Read the model definition and answer for the solid it produces. Units are mm, in the model's axes. Face numbers are marked on the shaded views. A direction names the side the tool comes from. Coordinates: 2 decimals unless noted, no trailing zeros. Write each loop counter-clockwise with the first axis right and the second up, starting at its lowest first coordinate (ties: lowest second). Pieces come first, ordered by that corner, then holes.
1) Find the intervals of material crossed by line 1 (X direction, y = 1.3, z = 40); line 2 (Z direction, x = 14.5, y = -26.5); line 3 (X direction, y = -19, z = -13), in increasing order.
2) The part is cut by section A-A (y = -37.5). Determine the outline of the cut face in (x, z).
3) The part is cut by section C-C (z = 9). Determine the outline of the cut face in (x, y), then the cut area to 3 significant figures.
4) The part is cut by section D-D (z = 18). Determine the outline of the cut face in (x, y), then the cut area to 3 significant figures.
5) Each of these flat-tipped pins is pushed along its axis until it touches: pin 1 Ø23 at (y, z) = (-34.5, -18) entering from -X; pin 2 Ø25 at (x, y) = (33, -26.5) entering from +Z; pin 3 Ø13.5 at (x, z) = (25, 24.5) entering from -Y; pin 4 Ø1.5 at (x, z) = (24.5, 1.5) entering from -Y. Where does it stop, or does it pass through?
6) Determine the mould class of the marked faces 1, 2, 3 and 4 for opening direction Z: +Z half, -Z half, draft (parallel to the pull), parting line (faces both ways), or undercut.
7) Which of the six approach directions +Z, -Z, +X, -X, +Y, -Y give full straight-line access (tool end or side, diameter ignored) to the marked faces 5, 6, 7 and 8?
8) The part is cut by section B-B (x = 25). Determine the outline of the cut face in (y, z), then the cut area to 3 significant figures.
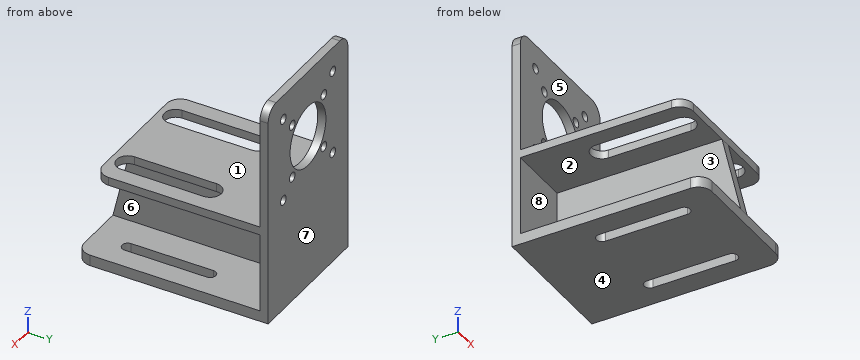
Autodesk Fusion 360 part; units mm, degrees
sketch "Sketch1" plane through (0, 0, 0) normal (0, 1, 0) x (1, 0, 0)
  line L0 (0, 0) -> (50, 0)
  line L1 (50, 0) -> (50, -49)
  line L2 (50, -49) -> (0, -49)
  line L3 (0, -49) -> (0, 0)
  line L4 (0, -24.5) -> (50, -24.5) construction
  line L5 (25, -49) -> (25, 0) construction
  circle A0 centre (25, -24.5) radius 11.25
  circle A1 centre (25, -24.5) radius 14 construction
  line L6 (0, -49) -> (0, -40) construction
  line L7 (0, -40) -> (9.5, -40) construction
  circle A2 centre (9.5, -40) radius 1.75
  line L8 (9.5, -40) -> (25, -24.5) construction
  circle A3 centre (15.1005, -34.3995) radius 1.75
  circle A4 centre (40.5, -40) radius 1.75
  circle A5 centre (34.8995, -34.3995) radius 1.75
  circle A6 centre (40.5, -9) radius 1.75
  circle A7 centre (34.8995, -14.6005) radius 1.75
  circle A8 centre (15.1005, -14.6005) radius 1.75
  circle A9 centre (9.5, -9) radius 1.75
  line L9 (0, -49) -> (5, -49)
  line L10 (5, -49) -> (5, -44) construction
  line L11 (5, -44) -> (0, -44) construction
  line L12 (0, -44) -> (0, -49)
  arc A10 (0, -44) -> (5, -49) centre (5, -44) ccw
  arc A11 (45, -49) -> (50, -44) centre (45, -44) ccw
  dimension "d1" = 50
  dimension "d2" = 49
  dimension "d3" = 22.5
  dimension "d4" = 28
  dimension "d5" = 9
  dimension "d6" = 9.5
  dimension "d7" = 3.5
  dimension "d8" = 3.5
  dimension "d11" = 5
  dimension "d12" = 5
extrude "Extrude2" add sketch "Sketch1" along normal blind 3 contours L0 L1 L2 L3 A10 A11
sketch "Sketch2" plane through (0, 0, 0) normal (0, 0, 1) x (1, 0, 0)
  line L0 (0, 3) -> (50, 3)
  line L1 (50, 3) -> (50, -67)
  line L2 (50, -67) -> (0, -67)
  line L3 (0, -67) -> (0, 3)
  line L4 (25, -67) -> (25, 3) construction
  line L5 (0, -67) -> (10, -67) construction
  line L6 (10, -67) -> (10, -54) construction
  line L7 (10, -54) -> (7.9, -54) construction
  line L8 (7.9, -54) -> (12.1, -54)
  line L9 (12.1, -54) -> (12.1, -24)
  line L10 (12.1, -24) -> (7.9, -24)
  line L11 (7.9, -24) -> (7.9, -54)
  arc A0 (7.9, -54) -> (12.1, -54) centre (10, -54) ccw
  arc A1 (12.1, -24) -> (7.9, -24) centre (10, -24) ccw
  arc A2 (37.9, -54) -> (42.1, -54) centre (40, -54) ccw
  line L12 (37.9, -54) -> (37.9, -24)
  line L13 (42.1, -24) -> (42.1, -54)
  arc A3 (42.1, -24) -> (37.9, -24) centre (40, -24) ccw
  line L14 (0, 0) -> (50, 0)
  point P0 (0, 3)
  dimension "d15" = 70
  dimension "d16" = 10
  dimension "d17" = 13
  dimension "d18" = 2.1
  dimension "d19" = 4.2
  dimension "d20" = 30
extrude "Extrude6" add sketch "Sketch2" against normal blind 32.6
extrude "Extrude7" cut sketch "Sketch2" against normal blind 28.6 contours L1 L2 L3 L14
ref_plane "WorkPlane1" through (25, -32, 5.7) normal (1, 0, 0) x (0, 0, -1)
sketch "Sketch6" plane through (25, -32, 5.7) normal (1, 0, 0) x (0, 1, 0)
  line L0 (32, -34.3) -> (-35, -34.3)
  line L1 (-35, -34.3) -> (-35, -5.3)
  line L2 (-35, -5.3) -> (32, -5.3)
  line L3 (32, -5.3) -> (32, -34.3)
  point P0 (32, -34.3)
  dimension "d48" = 67
  dimension "d49" = 29
sketch "Sketch10" plane through (0, 0, 0) normal (0, -1, 0) x (1, 0, 0)
  circle A0 centre (25, 24.5) radius 11.25
  circle A1 centre (9.5, 40) radius 1.75
  circle A2 centre (40.5, 40) radius 1.75
  circle A3 centre (15.1005, 34.3995) radius 1.75
  circle A4 centre (34.8995, 34.3995) radius 1.75
  circle A5 centre (40.5, 9) radius 1.75
  circle A6 centre (34.8995, 14.6005) radius 1.75
  circle A7 centre (15.1005, 14.6005) radius 1.75
  circle A8 centre (9.5, 9) radius 1.75
  arc A9 (5, 49) -> (0, 44) centre (5, 44) ccw
  line L0 (0, 44) -> (0, -28.6)
  line L1 (0, -28.6) -> (50, -28.6)
  line L2 (50, -28.6) -> (50, 44)
  arc A10 (50, 44) -> (45, 49) centre (45, 44) ccw
  line L3 (45, 49) -> (5, 49)
  line L4 (25, 24.5) -> (25, 3.4) construction
  dimension "d71" = 21.1
extrude "Extrude15" add sketch "Sketch6" along normal blind 2 and the other way blind 2
sketch "Sketch11" plane through (0, 0, 0.4) normal (0, 0, 1) x (-1, 0, 0)
  line L0 (-23, 67) -> (-27, 67)
  line L1 (-27, 67) -> (-27, 0)
  line L2 (-27, 0) -> (-23, 0)
  line L3 (-23, 0) -> (-23, 67)
  line L4 (0, 0) -> (-50, 0)
  line L5 (-50, 0) -> (-50, 60.1926)
  line L6 (-50, 60.1926) -> (0, 60.1926)
  line L7 (0, 60.1926) -> (0, 0)
  line L8 (-50, -3) -> (-50, 67)
  line L9 (-7.9, 24) -> (-5.9, 24)
  line L10 (-5.9, 24) -> (-14.1, 24)
  line L11 (-14.1, 24) -> (-14.1, 54)
  line L12 (-14.1, 54) -> (-5.9, 54)
  line L13 (-5.9, 54) -> (-5.9, 24)
  arc A0 (-5.9, 54) -> (-14.1, 54) centre (-10, 54) ccw
  arc A1 (-14.1, 24) -> (-5.9, 24) centre (-10, 24) ccw
  line L14 (-25, 67) -> (-25, 0)
  line L15 (-25, 60.1926) -> (-25, 53.1429)
  line L16 (-35.9, 24) -> (-35.9, 54)
  line L17 (-44.1, 54) -> (-44.1, 24)
  arc A2 (-35.9, 54) -> (-44.1, 54) centre (-40, 54) ccw
  arc A3 (-44.1, 24) -> (-35.9, 24) centre (-40, 24) ccw
  point P0 (-7.9, 24)
  dimension "d76" = 2
  dimension "d77" = 8.2
extrude "Extrude16" add sketch "Sketch11" along normal blind 3 contours L3 L4 L6 L7 | L2 L3 L4 L6 L14 L15 | L1 L2 L4 L6 L14 L15 | L1 L4 L5 L6 L8
sketch "Sketch12" plane through (27, 0, 0) normal (1, 0, 0) x (0, 1, 0)
  line L0 (0, 0.4) -> (-60.1926, 0.4)
  line L1 (-60.1926, 0.4) -> (-67, 0.4)
  line L2 (-67, 0.4) -> (-67, -28.6)
  line L3 (-67, -28.6) -> (0, -28.6)
  line L4 (0, -28.6) -> (0, 0.4)
  line L5 (-60.1926, 0.4) -> (-67, -28.6)
  line L6 (-67, 0.4) -> (-60.1926, 0.4)
extrude "Extrude17" cut sketch "Sketch12" against normal blind 8 contours L1 L2 L5 L6
fillet "Fillet3" radius 5 4 edges at (0, -60.1926, 1.9) (0, -67, -30.6) (50, -67, -30.6) (50, -60.1926, 1.9)
Reported:
1. line 1: x = 0 to 7.75, 11.25 to 38.75, 42.25 to 50
1. line 2: z = -32.6 to -28.6, 0.4 to 3.4
1. line 3: x = 23 to 27
2. outline: (0, -32.6) - (7.9, -32.6) - (7.9, -28.6) - (0, -28.6) - close; (0, 0.4) - (5.9, 0.4) - (5.9, 3.4) - (0, 3.4) - close; (12.1, -32.6) - (37.9, -32.6) - (37.9, -28.6) - (27, -28.6) - (27, 0.4) - (35.9, 0.4) - (35.9, 3.4) - (14.1, 3.4) - (14.1, 0.4) - (23, 0.4) - (23, -28.6) - (12.1, -28.6) - close; (42.1, -32.6) - (50, -32.6) - (50, -28.6) - (42.1, -28.6) - close; (44.1, 0.4) - (50, 0.4) - (50, 3.4) - (44.1, 3.4) - close
3. outline: (0, 0) - (7.75, 0) - (7.75, 3) - (0, 3) - close; (11.25, 0) - (38.75, 0) - (38.75, 3) - (11.25, 3) - close; (42.25, 0) - (50, 0) - (50, 3) - (42.25, 3) - close
3. area: 129 mm2
4. outline: (0, 0) - (15.82, 0) - (15.82, 3) - (0, 3) - close; (34.18, 0) - (50, 0) - (50, 3) - (34.18, 3) - close
4. area: 94.9 mm2
5. pin 1: stops at x = 0
5. pin 2: stops at z = 3.4
5. pin 3: passes through
5. pin 4: stops at y = -60.19
6. face 1: +Z half
6. face 2: undercut
6. face 3: undercut
6. face 4: -Z half
7. face 5: +Z, +X, -X, -Y
7. face 6: +X, -Y
7. face 7: +Z, -Z, +X, -X, +Y
7. face 8: -X, -Y
8. outline: (-67, -32.6) - (3, -32.6) - (3, 13.25) - (0, 13.25) - (0, 3.4) - (-60.19, 3.4) - (-60.19, 0.4) - (-67, -28.6) - close; (0, 35.75) - (3, 35.75) - (3, 49) - (0, 49) - close
8. area: 2,470 mm2
